```python
from build123d import *

# Parameters (mm, degrees)
SKETCH1_W           = 6.3
SKETCH1_H           = 6.3
BOSS_EXTRUDE1_DEPTH = 10.43
SKETCH2_R           = 3.15
BOSS_EXTRUDE2_DEPTH = 7.9
SKETCH3_R           = 0.475
BOSS_EXTRUDE3_DEPTH = 3.1


with BuildPart() as part:
    # Sketch1 → Boss-Extrude1 (new body)
    with BuildSketch(Plane(origin=(0, 0, 0), x_dir=(1, 0, 0), z_dir=(0, 1, 0))):
        Rectangle(SKETCH1_W, SKETCH1_H)
    extrude(amount=BOSS_EXTRUDE1_DEPTH)

    # Sketch2 → Boss-Extrude2 (add)
    with BuildSketch(Plane(origin=(0, 0, -3.15), x_dir=(-1, 0, 0), z_dir=(0, 0, -1))):
        with Locations((0, 7.029219023)):
            Circle(SKETCH2_R)
    extrude(amount=BOSS_EXTRUDE2_DEPTH)

    # Sketch3 → Boss-Extrude3 (add)
    with BuildSketch(Plane(origin=(0, 0, 0), x_dir=(-1, 0, 0), z_dir=(0, -1, 0))):
        Circle(SKETCH3_R)
        with Locations((2.675, -2.675)):
            Circle(SKETCH3_R)
        with Locations((-2.675, -2.675)):
            Circle(SKETCH3_R)
        with Locations((2.675, 2.66524354)):
            Circle(SKETCH3_R)
        with Locations((-2.675, 2.66524354)):
            Circle(SKETCH3_R)
    extrude(amount=BOSS_EXTRUDE3_DEPTH)


solid = part.part
```
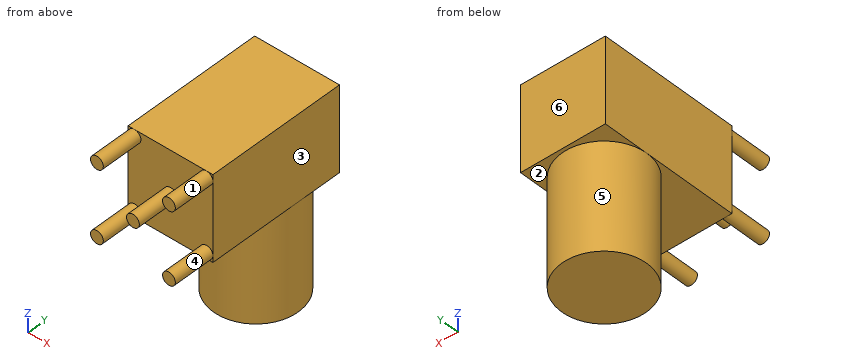
Part model, mm, in its own coordinate system. Face numbers are marked on the shaded views. A direction names the side the tool comes from. Give positions to 0.01 mm unless a question says otherwise; leave off trailing zeros. Write each loop counter-clockwise with the first axis right and the second up, starting at its lowest first coordinate (ties: lowest second). Pieces come first, ordered by that corner, then holes. Notation, with made-up numbers: (-34, 10.25) -> (0, 10.25) arc R33 cw to (0, 39.25) -> close; hole circle Ø9 at (-14.5, 27). An arc over 180 degrees is marked (long way). Put each result on its own line as item: value. Start each with the question number.
Item 1: Which spindle directions (+Z, -Z, +X, -X, +Y, -Y) get a long thin tool onto all of the face, cutting with end or side? Do the marked faces 4, 5 and 6. Say none if no direction does.
Item 2: Cut at C-C (y = 1.5). List the corners of the cut face in (x, z).
Item 3: Cut at A-A (z = 0). List the corners of the cut face in (x, y) (3 decimals), then the cut area to 3 significant figures.
Item 4: Pin check, flat tip, straight feed: pin 1 Ø2 at (x, z) = (2.5, -4.5) entering from +Y. Stop position of the tip, or through.
Item 5: Pull direction Z, two halves, no side cores. Call the marked faces 1, 2 and 3: pulls with the +Z half, pulls with the -Z half, needs draft (parallel to the pull), parting line crosses it, or undercut.
Item 6: Wall check: L1, parallel to Y at x = -0.25, z = 1.25; L2, parallel to Z at x = -2.5, y = 0.25; L3, parallel to Z at x = 3, y = -2. Give the ranges that are in metal, low to high. Write a range as [from, to].
Item 7: Cut at B-B (x = 0). List the corners of the cut face in (y, z) (3 decimals), then the cut area to 3 significant figures.
Item 8: Cut at D-D (x = 1.25). List the corners of the cut face in (y, z), then the cut area to 3 significant figures.
Answer list:
1. face 4: -Y
1. face 5: -Z
1. face 6: +Z, -Z, +X, -X, +Y
2. outline: (-3.15, -3.15) -> (3.15, -3.15) -> (3.15, 3.15) -> (-3.15, 3.15) -> close
3. outline: (-3.15, 0) -> (-0.475, 0) -> (-0.475, -3.1) -> (0.475, -3.1) -> (0.475, 0) -> (3.15, 0) -> (3.15, 10.43) -> (-3.15, 10.43) -> close
3. area: 68.7 mm2
4. pin 1: stops at y = 9.8
5. face 1: undercut
5. face 2: pulls with the -Z half
5. face 3: needs draft
6. L1: y = [0, 10.43]
6. L2: z = [-3.15, 3.15]
6. L3: z = [-3.01, -2.32], [2.33, 3.02]
7. outline: (-3.1, -0.475) -> (0, -0.475) -> (0, -3.15) -> (3.879, -3.15) -> (3.879, -11.05) -> (10.179, -11.05) -> (10.179, -3.15) -> (10.43, -3.15) -> (10.43, 3.15) -> (0, 3.15) -> (0, 0.475) -> (-3.1, 0.475) -> close
7. area: 118 mm2
8. outline: (0, -3.15) -> (4.14, -3.15) -> (4.14, -11.05) -> (9.92, -11.05) -> (9.92, -3.15) -> (10.43, -3.15) -> (10.43, 3.15) -> (0, 3.15) -> close
8. area: 111 mm2
